```python
from build123d import *

# Parameters (mm, degrees)
F1_ANGLE = 90
F2_DEPTH = 7
F3_DEPTH = 7
F4_DEPTH = 7
F5_T     = -1.5
F6_R     = 1


with BuildPart() as f1:
    # F0 (on Top) → F1 (revolve)
    with BuildSketch(Plane.XY):
        with BuildLine():
            Line((-13, 0), (0, 0))
            Line((0, 0), (0, 13))
            ThreePointArc((0, 13), (-9.1923881554, 9.1923881554), (-13, 0))
        make_face()
    revolve(axis=Axis((0, 6.5, 0), (0, 1, 0)), revolution_arc=F1_ANGLE)

    # F2 (add): a face of the model
    f2_faces = [f1.faces().sort_by_distance(p)[0] for p in [
        (0, 5.5173713605, 5.5173713605),
    ]]
    extrude(f2_faces, amount=F2_DEPTH)

    # F3 (add): a face of the model
    f3_faces = [f1.faces().sort_by_distance(p)[0] for p in [
        (-1.8496808576, 5.9170419058, 0),
    ]]
    extrude(f3_faces, amount=F3_DEPTH)

    # F4 (add): a face of the model
    f4_faces = [f1.faces().sort_by_distance(p)[0] for p in [
        (-2.29243693, 0, 2.29243693),
    ]]
    extrude(f4_faces, amount=F4_DEPTH)

    # F5
    f5_openings = [f1.faces().sort_by_distance(p)[0] for p in [
        (7, 2.292437, 2.292437),
        (-2.292437, 2.292437, -7),
        (-2.292437, -7, 2.292437),
    ]]
    offset(amount=F5_T, openings=f5_openings)

    # F6
    f6_edges = [f1.edges().sort_by_distance(p)[0] for p in [
        (7, -7, 12.25),
        (7, 12.25, -7),
        (-12.25, -7, -7),
    ]]
    fillet(f6_edges, radius=F6_R)


solid = f1.part
```
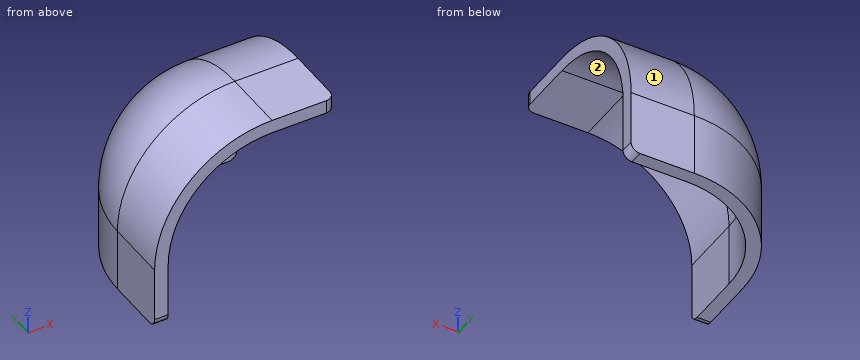
Geometry check sheet. Reference: the model listing, model coordinates, mm. Face numbers are marked on the shaded views. A direction names the side the tool comes from. Coordinates: 2 decimals unless noted, no trailing zeros. Order: outer loops, then holes, each group sorted by start corner. A loop starts at its lowest first (then second) coordinate and runs counter-clockwise, first axis right, second up.
Item 1: Section check C-C (z = 12.25). Enter the section's corners in (x, y), plus the area to 3 significant figures.
Item 2: Tool access check on the marked faces 1 and 2. Record the directions out of +Z, -Z, +X, -X, +Y, -Y that give a thin tool (end or side, any length) a straight path to the whole face; none if there is none.
Item 3: Scan lines: line 1 along Y through (x, z) = (0.25, -5.5); line 2 along X through (y, z) = (-5, -4.25); line 3 along Z through (x, y) = (-8.25, 3.5). Record each from-to range of solid material in increasing order.
Item 4: Section check B-B (x = 3.75). Enter the section's corners in (y, z).
Item 5: Section check A-A (y = -5.25). Enter the section's corners in (x, z).
Item 6: Depth check by flat-ended pin: pin 1 (1.5 mm diameter, centred on x = -3, z = -1.5, fed in from -Y); pin 2 (8 mm diameter, centred on y = 9.5, z = 3, fed in from -X); pin 3 (2 mm diameter, centred on y = -2, z = -3.5, fed in from +X); pin 4 (5 mm diameter, centred on x = 0, z = 2, fed in from +Y). Enter the tip coordinate at first touch or a pass-through.
Check sheet entries:
1. outline: (-4.35, -7) - (6, -7) arc R1 ccw to (7, -6) - (7, 4.35) - (0, 4.35) arc R4.35 ccw to (-4.35, 0) - close
1. area: 125 mm2
2. face 1: +Z, +X, -X, +Y
2. face 2: -Z, +X, -Y
3. line 1: y = 11.5 to 13
3. line 2: x = -13 to -11.5
3. line 3: z = 7.21 to 9.42
4. outline: (-7, 11.5) - (0, 11.5) arc R11.5 cw to (11.5, 0) - (11.5, -7) - (13, -7) - (13, 0) arc R13 ccw to (0, 13) - (-7, 13) - close
5. outline: (-13, -7) - (-11.5, -7) - (-11.5, 0) arc R11.5 cw to (0, 11.5) - (7, 11.5) - (7, 13) - (0, 13) arc R13 ccw to (-13, 0) - close
6. pin 1: stops at y = 10.87
6. pin 2: stops at x = -11.55
6. pin 3: stops at x = -11.5
6. pin 4: stops at y = 13
